Geometry: see drawing. Coordinates: mm, zero at the bounding-box minimum. A direction names the side the tool comes from. Coordinates: 2 decimals unless noted, no trailing zeros. Write each loop counter-clockwise with the first axis right and the second up, starting at its lowest first coordinate (ties: lowest second). Pieces come first, ordered by that corner, then holes. Notation, with made-up numbers: (-34, 11.25) - (3, 11.25) arc R8 ccw to (3, 26.25) - close; hole circle Ø8 at (1, 0.25). An arc over 180 degrees is marked (long way). One line per question, with ' | ' between items. Start each with the question number.
1) Line query: line 1 (X direction, y = 22, z = 2.8) (1 decimal); line 2 (Y direction, x = 15.75, z = 0.4) (1 decimal); line 3 (Y direction, x = 7.25, z = 2) (1 decimal). Output: solid intervals per line, ascending.
2) First-contact query: P1, Ø6.5, axis at x = 17.12, y = 26.54, coming from the +Z side; P2, Ø1, axis at x = 16, z = 0.5, coming from the -Y side; P3, Ø1.5, axis at x = 7, z = 2.5, coming from the -Y side. Flat tips, straight axial feed; report the tip coordinate or a pass-through.
3) Draft query along X for the marked faces 1, 2, 3 and 4. Return one class per face: released by +X, released by -X, zero draft, split by the parting line, or undercut.
4) Section query D-D on y = 22.5. Return loops of the section in (x, z) (1 decimal).
5) Section query B-B on y = 8. Return loops of the section in (x, z) (1 decimal).
6) Section query A-A on x = 8. Return loops of the section in (y, z) (1 decimal).
7) Section query C-C on z = 1.25. Give the number of separate pieces and of enclosed holes in the cut face, and give its area (3 significant figures).
8) Reachability of the marked faces 5 and 6 from +Z, -Z, +X, -X, +Y, -Y: full face, straight path, thin tool, end or side. Return the list, or none.
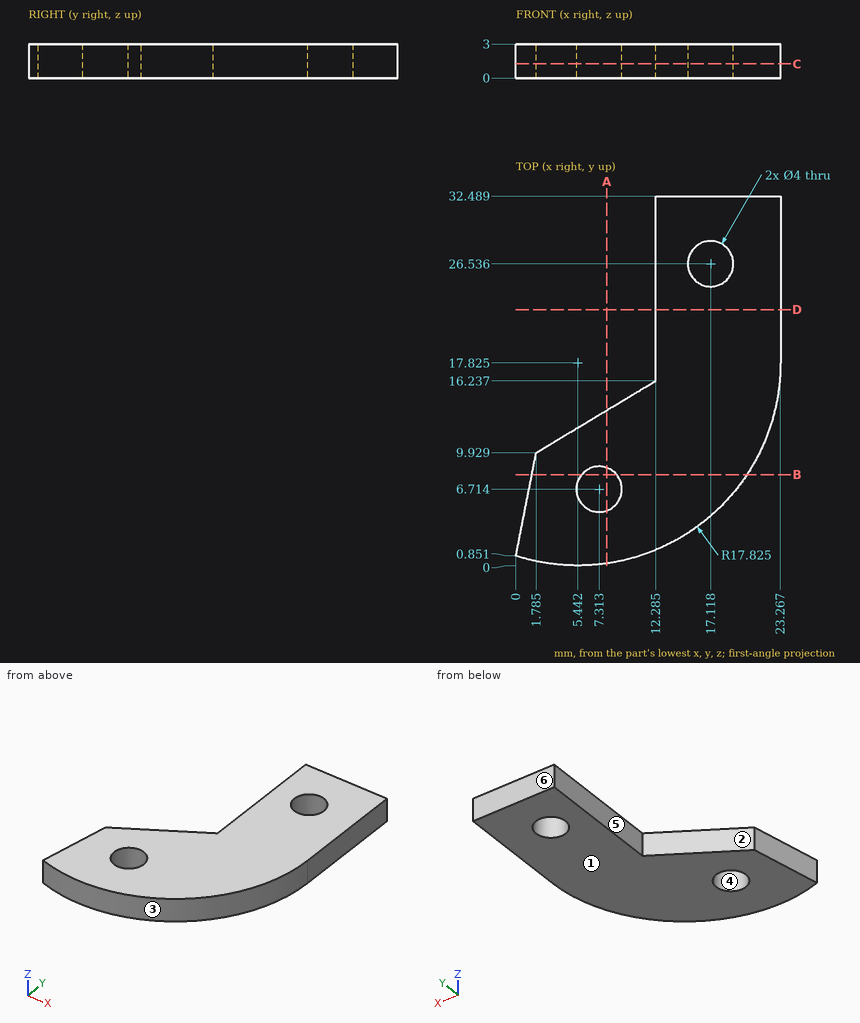
Answer key:
1) line 1: 12.3 to 23.3 | line 2: 3.3 to 25.1, 28 to 32.5 | line 3: 0.1 to 4.7, 8.7 to 13.2
2) P1: z = 3 | P2: y = 3.11 | P3: y = 0.02
3) face 1: zero draft | face 2: released by -X | face 3: split by the parting line | face 4: undercut
4) outline: (12.3, 0) - (23.3, 0) - (23.3, 3) - (12.3, 3) - close
5) outline: (1.4, 0) - (5.8, 0) - (5.8, 3) - (1.4, 3) - close; (8.8, 0) - (20.3, 0) - (20.3, 3) - (8.8, 3) - close
6) outline: (0.2, 0) - (4.8, 0) - (4.8, 3) - (0.2, 3) - close; (8.6, 0) - (13.7, 0) - (13.7, 3) - (8.6, 3) - close
7) separate pieces: 1 | enclosed holes: 2 | area: 409 mm²
8) face 5: +Z, -Z, -X, +Y | face 6: +Z, -Z, +X, -X, +Y
